```python
from build123d import *

# Parameters (mm, degrees)
SKETCH1_W               = 184
SKETCH1_H               = 15
BOSS_EXTRUDE1_DEPTH     = 6
CUT_EXTRUDE1_DEPTH      = 141.246944523
CUT_EXTRUDE1_DEPTH_BACK = 141.246944523
SKETCH2_W               = 6.5
SKETCH2_H               = 5.5
CUT_EXTRUDE2_DEPTH      = 141.246944523
CUT_EXTRUDE2_DEPTH_BACK = 141.246944523
SKETCH3_W               = 6.5
SKETCH3_H               = 5.5
CUT_EXTRUDE3_DEPTH      = 141.246944523
CUT_EXTRUDE3_DEPTH_BACK = 141.246944523
SKETCH4_W               = 6.5
SKETCH4_H               = 5.5
CUT_EXTRUDE4_DEPTH      = 141.246944523
CUT_EXTRUDE4_DEPTH_BACK = 141.246944523
SKETCH5_W               = 6.5
SKETCH5_H               = 5.5
CUT_EXTRUDE5_DEPTH      = 141.246944523
CUT_EXTRUDE5_DEPTH_BACK = 4
SKETCH8_W               = 184
SKETCH8_H               = 11.3
SKETCH9_W               = 12
SKETCH9_H               = 7.5
SKETCH9_W_2             = 12.5
SKETCH9_H_2             = 4
CUT_EXTRUDE6_DEPTH      = 1.5
SKETCH10_W              = 12.5
SKETCH10_H              = 4
CUT_EXTRUDE7_DEPTH      = 1.5
CUT_EXTRUDE8_DEPTH      = 184
SKETCH13_W              = 0.5
SKETCH13_H              = 10
CUT_EXTRUDE9_DEPTH      = 0.6
FILLET1_R               = 0.25
FILLET2_R               = 0.25
SKETCH16_W              = 15
SKETCH16_H              = 0.5
BOSS_EXTRUDE2_DEPTH     = 0.75
FILLET3_R               = 0.5
FILLET4_R               = 0.25
SKETCH17_W              = 15
SKETCH17_H              = 0.5
BOSS_EXTRUDE3_DEPTH     = 0.75
FILLET5_R               = 0.5
FILLET6_R               = 0.25
LPATTERN1_COUNT         = 3
LPATTERN1_PITCH         = 47
LPATTERN2_COUNT         = 3
LPATTERN2_PITCH         = 47
FILLET7_R               = 0.5
FILLET8_R               = 0.25
FILLET9_R               = 0.5
FILLET10_R              = 0.25
CHAMFER1_SIZE           = 0.4
CHAMFER2_SIZE           = 0.4
CHAMFER3_SIZE           = 0.4
CHAMFER5_SIZE           = 0.4


# Some blends are built 0.0001 mm under size
with BuildPart() as part:
    # Sketch1 → Boss-Extrude1 (new body)
    with BuildSketch(Plane.XY):
        with Locations((-45.75, 18.154296875)):
            Rectangle(SKETCH1_W, SKETCH1_H)
    extrude(amount=BOSS_EXTRUDE1_DEPTH)

    # Sketch2 → Cut-Extrude1 (cut, two sides: drawn at the far end of the back side and taken through both)
    with BuildSketch(Plane.XY.offset(6).offset(-CUT_EXTRUDE1_DEPTH_BACK)):
        with Locations((-126.4, 18.154296875)):
            Rectangle(SKETCH2_W, SKETCH2_H)
    extrude(amount=CUT_EXTRUDE1_DEPTH + CUT_EXTRUDE1_DEPTH_BACK, mode=Mode.SUBTRACT)

    # Sketch3 → Cut-Extrude2 (cut, two sides: drawn at the far end of the back side and taken through both)
    with BuildSketch(Plane.XY.offset(6).offset(-CUT_EXTRUDE2_DEPTH_BACK)):
        with Locations((-103.35, 18.154296875)):
            Rectangle(SKETCH3_W, SKETCH3_H)
    extrude(amount=CUT_EXTRUDE2_DEPTH + CUT_EXTRUDE2_DEPTH_BACK, mode=Mode.SUBTRACT)

    # Sketch4 → Cut-Extrude3 (cut, two sides: drawn at the far end of the back side and taken through both)
    with BuildSketch(Plane.XY.offset(6).offset(-CUT_EXTRUDE3_DEPTH_BACK)):
        with Locations((-80.3, 18.154296875)):
            Rectangle(SKETCH4_W, SKETCH4_H)
    extrude(amount=CUT_EXTRUDE3_DEPTH + CUT_EXTRUDE3_DEPTH_BACK, mode=Mode.SUBTRACT)

    # Sketch5 → Cut-Extrude4 (cut, two sides: drawn at the far end of the back side and taken through both)
    with BuildSketch(Plane.XY.offset(6).offset(-CUT_EXTRUDE4_DEPTH_BACK)):
        with Locations((-57.25, 18.154296875)):
            Rectangle(SKETCH5_W, SKETCH5_H)
        with Locations((-34.2, 18.154296875)):
            Rectangle(SKETCH5_W, SKETCH5_H)
        with Locations((-11.15, 18.154296875)):
            Rectangle(SKETCH5_W, SKETCH5_H)
        with Locations((11.9, 18.154296875)):
            Rectangle(SKETCH5_W, SKETCH5_H)
        with Locations((34.95, 18.154296875)):
            Rectangle(SKETCH5_W, SKETCH5_H)
    extrude(amount=CUT_EXTRUDE4_DEPTH + CUT_EXTRUDE4_DEPTH_BACK, mode=Mode.SUBTRACT)

    # Sketch8 → Cut-Extrude5 (cut, two sides: drawn at the far end of the back side and taken through both)
    with BuildSketch(Plane.XY.offset(6).offset(-CUT_EXTRUDE5_DEPTH_BACK)):
        with Locations((-45.75, 18.154296875)):
            Rectangle(SKETCH8_W, SKETCH8_H)
    extrude(amount=CUT_EXTRUDE5_DEPTH + CUT_EXTRUDE5_DEPTH_BACK, mode=Mode.SUBTRACT)

    # Sketch9 → Cut-Extrude6 (cut)
    with BuildSketch(Plane.XY.offset(2)):
        with Locations((-57.75, 18.154296875)):
            Rectangle(SKETCH9_W, SKETCH9_H)
        with Locations((-33.95, 18.154296875)):
            Rectangle(SKETCH9_W, SKETCH9_H)
        with Locations((-125.9, 18.154296875)):
            Rectangle(SKETCH9_W, SKETCH9_H)
        with Locations((-11.15, 18.154296875)):
            Rectangle(SKETCH9_W_2, SKETCH9_H_2)
        with Locations((11.9, 18.154296875)):
            Rectangle(SKETCH9_W_2, SKETCH9_H_2)
        with Locations((34.7, 18.154296875)):
            Rectangle(SKETCH9_W, SKETCH9_H)
    extrude(amount=-CUT_EXTRUDE6_DEPTH, mode=Mode.SUBTRACT)

    # Sketch10 → Cut-Extrude7 (cut)
    with BuildSketch(Plane.XY.offset(2)):
        with Locations((-80.3, 18.154296875)):
            Rectangle(SKETCH10_W, SKETCH10_H)
        with Locations((-103.35, 18.154296875)):
            Rectangle(SKETCH10_W, SKETCH10_H)
    extrude(amount=-CUT_EXTRUDE7_DEPTH, mode=Mode.SUBTRACT)

    # Sketch12 → Cut-Extrude8 (cut)
    with BuildSketch(Plane(origin=(46.25, 0, 0), x_dir=(0, 0, -1), z_dir=(1, 0, 0))):
        Polygon((-6, 25.654296875), (-6, 24.654296875), (-5, 25.654296875), align=None)
        Polygon((-6, 10.654296875), (-5, 10.654296875), (-6, 11.654296875), align=None)
    extrude(amount=-CUT_EXTRUDE8_DEPTH, mode=Mode.SUBTRACT)

    # Sketch13 → Cut-Extrude9 (cut)
    with BuildSketch(Plane(origin=(0, 0, 0), x_dir=(-1, 0, 0), z_dir=(0, 0, -1))):
        with Locations((135.5, 18.154296875)):
            Rectangle(SKETCH13_W, SKETCH13_H)
    extrude(amount=-CUT_EXTRUDE9_DEPTH, mode=Mode.SUBTRACT)

    # Fillet1
    fillet1_edges = [part.edges().sort_by_distance(p)[0] for p in [
        (-135.75, 18.154296875, 0),
    ]]
    fillet(fillet1_edges, radius=FILLET1_R)

    # Fillet2
    fillet2_edges = [part.edges().sort_by_distance(p)[0] for p in [
        (-135.25, 18.154296875, 0.6),
        (-135.5, 23.154296875, 0.6),
        (-135.75, 18.154296875, 0.6),
        (-135.5, 13.154296875, 0.6),
    ]]
    fillet(fillet2_edges, radius=FILLET2_R - 0.0001)  # a hair under: the kernel refuses the full size

    # Sketch16 → Boss-Extrude2 (add)
    with BuildSketch(Plane.XZ.offset(-23.804296875)):
        with Locations((-115.25, 4)):
            Rectangle(SKETCH16_W, SKETCH16_H)
    boss_extrude2 = extrude(amount=BOSS_EXTRUDE2_DEPTH)

    # Fillet3
    fillet3_edges = [part.edges().sort_by_distance(p)[0] for p in [
        (-115.25, 23.054296875, 4.25),
    ]]
    fillet(fillet3_edges, radius=FILLET3_R - 0.0001)  # a hair under: the kernel refuses the full size

    # Fillet4
    # the kernel refuses this fillet: 0.25 mm, written as the material it takes off along each edge
    with BuildSketch(Plane(origin=(-124.517583763, 23.054296875, 3.75), x_dir=(0, 0.7070334884245003, 0.7071800663524687), z_dir=(1, 0, 0))) as fillet4_piece_1:
        with BuildLine():
            CenterArc((0.530239772, -0.176759658), FILLET4_R, 44.994478191, 179.999583317)
            Line((0.353444756, -0.35351803), (0.335765254, -0.371193867))
            Line((0.335765254, -0.371193867), (-0.017679502, -0.017675837))
            Line((-0.017679502, -0.017675837), (-0.017675837, 0.017679502))
            ThreePointArc((-0.017675837, 0.017679502), (-0.017605119, 0.017750205), (0.724712877, 0.017675966))
            Line((0.724712877, 0.017675966), (0.707033504, 0))
        make_face()
    extrude(amount=18.535167526, mode=Mode.SUBTRACT)

    # Sketch17 → Boss-Extrude3 (add)
    with BuildSketch(Plane(origin=(0, 12.504296875, 0), x_dir=(1, 0, 0), z_dir=(0, 1, 0))):
        with Locations((-115.25, -4)):
            Rectangle(SKETCH17_W, SKETCH17_H)
    boss_extrude3 = extrude(amount=BOSS_EXTRUDE3_DEPTH)

    # Fillet5
    fillet5_edges = [part.edges().sort_by_distance(p)[0] for p in [
        (-115.25, 13.254296875, 4.25),
    ]]
    fillet(fillet5_edges, radius=FILLET5_R - 0.0001)  # a hair under: the kernel refuses the full size

    # Fillet6
    # the kernel refuses this fillet: 0.25 mm, written as the material it takes off along each edge
    with BuildSketch(Plane(origin=(-105.982416233, 13.254296875, 3.75), x_dir=(0, -0.7070334900459336, 0.7071800647313715), z_dir=(-1, 0, 0))) as fillet6_piece_1:
        with BuildLine():
            CenterArc((0.530239774, -0.176759657), FILLET6_R, 44.994478059, 179.99958358)
            Line((0.353444758, -0.35351803), (0.335765256, -0.371193867))
            Line((0.335765256, -0.371193867), (-0.017679502, -0.017675837))
            Line((-0.017679502, -0.017675837), (-0.017675837, 0.017679502))
            ThreePointArc((-0.017675837, 0.017679502), (-0.017605119, 0.017750205), (0.724712878, 0.017675966))
            Line((0.724712878, 0.017675966), (0.707033505, 0))
        make_face()
    extrude(amount=18.535167534, mode=Mode.SUBTRACT)

    # LPattern1: Boss-Extrude3 ×3
    with Locations(*[(i * LPATTERN1_PITCH, 0, 0) for i in range(1, LPATTERN1_COUNT)]):
        add(boss_extrude3)

    # LPattern2: Boss-Extrude2 ×3
    with Locations(*[(i * LPATTERN2_PITCH, 0, 0) for i in range(1, LPATTERN2_COUNT)]):
        add(boss_extrude2)

    # Fillet7
    fillet7_edges = [part.edges().sort_by_distance(p)[0] for p in [
        (-68.25, 23.054296875, 4.25),
    ]]
    fillet(fillet7_edges, radius=FILLET7_R - 0.0001)  # a hair under: the kernel refuses the full size

    # Fillet8
    # the kernel refuses this fillet: 0.25 mm, written as the material it takes off along each edge
    with BuildSketch(Plane(origin=(-77.517583763, 23.054296875, 3.75), x_dir=(0, 0.7070334884245003, 0.7071800663524687), z_dir=(1, 0, 0))) as fillet8_piece_1:
        with BuildLine():
            CenterArc((0.530239772, -0.176759658), FILLET8_R, 44.994478191, 179.999583317)
            Line((0.353444756, -0.35351803), (0.335765254, -0.371193867))
            Line((0.335765254, -0.371193867), (-0.017679502, -0.017675837))
            Line((-0.017679502, -0.017675837), (-0.017675837, 0.017679502))
            ThreePointArc((-0.017675837, 0.017679502), (-0.017605119, 0.017750205), (0.724712877, 0.017675966))
            Line((0.724712877, 0.017675966), (0.707033504, 0))
        make_face()
    extrude(amount=18.535167526, mode=Mode.SUBTRACT)

    # Fillet9
    fillet9_edges = [part.edges().sort_by_distance(p)[0] for p in [
        (-68.25, 13.254296875, 4.25),
    ]]
    fillet(fillet9_edges, radius=FILLET9_R - 0.0001)  # a hair under: the kernel refuses the full size

    # Fillet10
    # the kernel refuses this fillet: 0.25 mm, written as the material it takes off along each edge
    with BuildSketch(Plane(origin=(-58.982416233, 13.254296875, 3.75), x_dir=(0, -0.7070334916347167, 0.7071800631429177), z_dir=(-1, 0, 0))) as fillet10_piece_1:
        with BuildLine():
            CenterArc((0.530239775, -0.176759657), FILLET10_R, 44.994477931, 179.999583837)
            Line((0.353444759, -0.35351803), (0.335765258, -0.371193867))
            Line((0.335765258, -0.371193867), (-0.017679502, -0.017675837))
            Line((-0.017679502, -0.017675837), (-0.017675837, 0.017679502))
            ThreePointArc((-0.017675837, 0.017679502), (-0.017605119, 0.017750205), (0.72471288, 0.017675966))
            Line((0.72471288, 0.017675966), (0.707033507, 0))
        make_face()
    extrude(amount=18.535167534, mode=Mode.SUBTRACT)

    # Chamfer1
    chamfer1_edges = [part.edges().sort_by_distance(p)[0] for p in [
        (-45.75, 25.654296875, 0),
        (-45.75, 10.654296875, 0),
    ]]
    chamfer(chamfer1_edges, length=CHAMFER1_SIZE)

    # Chamfer2
    chamfer2_edges = [part.edges().sort_by_distance(p)[0] for p in [
        (46.25, 18.154296875, 0),
        (-137.75, 18.154296875, 0),
    ]]
    chamfer(chamfer2_edges, length=CHAMFER2_SIZE)

    # Chamfer3
    chamfer3_edges = [part.edges().sort_by_distance(p)[0] for p in [
        (-137.75, 25.654296875, 2.7),
        (-137.75, 10.654296875, 2.7),
    ]]
    chamfer(chamfer3_edges, length=CHAMFER3_SIZE)

    # Chamfer5
    chamfer5_edges = [part.edges().sort_by_distance(p)[0] for p in [
        (46.25, 24.229296875, 6),
        (46.25, 25.654296875, 2.7),
        (46.25, 10.654296875, 2.7),
        (46.25, 12.079296875, 6),
        (46.25, 25.154296875, 5.5),
        (46.25, 11.154296875, 5.5),
    ]]
    chamfer(chamfer5_edges, length=CHAMFER5_SIZE)


solid = part.part
```
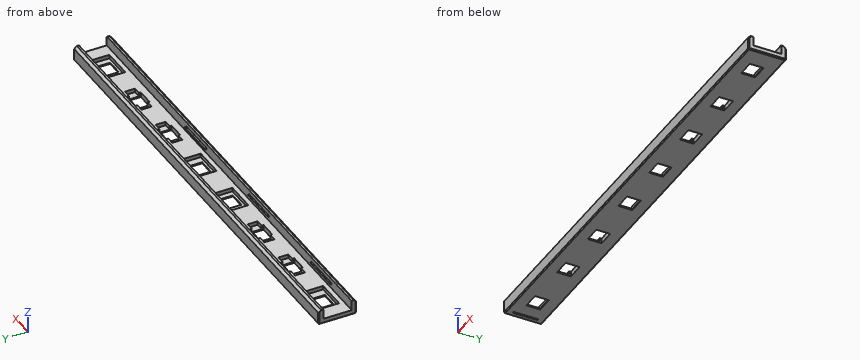
Input: part model. Units: mm. Frame: model coordinates. Coordinates: 2 decimals unless noted, no trailing zeros. Loops run counter-clockwise (first coordinate to the right, second up) from the corner with the lowest first, then second, coordinate; pieces in that order, holes last.
Q1. Section A-A, the plane x = -104. Return the cut outline in (y, z).
Results are:
outline: (10.65, 0.4) - (11.05, 0) - (15.4, 0) - (15.4, 2) - (12.5, 2) - (12.5, 6) - (11.65, 6) - (10.65, 5) - close; (20.9, 0) - (25.25, 0) - (25.65, 0.4) - (25.65, 5) - (24.65, 6) - (23.8, 6) - (23.8, 2) - (20.9, 2) - close
Q2. Line query: line 1 along Y through (x, z) = (-122, 1.25); line 2 along X through (y, z) = (21.75, 1.75); line 3 along Y through (x, z) = (-5, 1). Output: solid intervals per line, ascending.
Results are:
line 1: y = 10.65 to 14.4, 21.9 to 25.65
line 2: x = -137.75 to -131.9, -119.9 to -63.75, -51.75 to -39.95, -27.95 to 28.7, 40.7 to 46.25
line 3: y = 10.65 to 16.15, 20.15 to 25.65
Q3. Contact query for flat-ended pins moving along their axis: pin 1 (0.8 mm diameter, centred on x = -18, y = 13, fed in from +Z); pin 2 (2 mm diameter, centred on y = 14.5, z = 3.5, fed in from -X); pin 3 (2.5 mm diameter, centred on x = 16, y = 18, fed in from +Z). Output: stop coordinate, or through.
Results are:
pin 1: stops at z = 4.25
pin 2: passes through
pin 3: stops at z = 0.5
